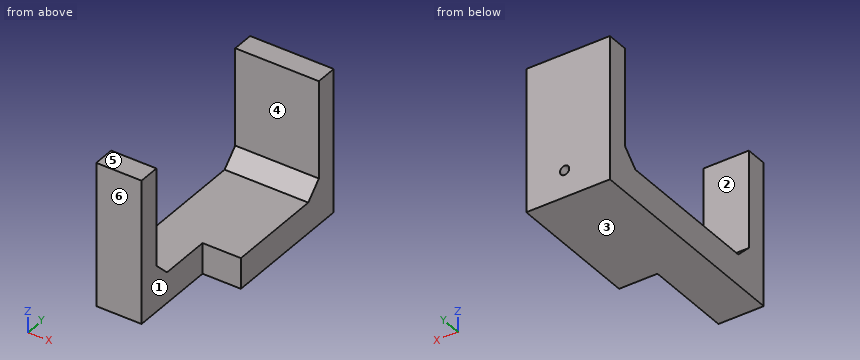
```python
from build123d import *

# Parameters (mm, degrees)
SKETCH026_W     = 10.9
SKETCH026_H     = 29
PAD009_DEPTH    = 4
SKETCH027_W     = 9
SKETCH027_H     = 14
POCKET015_DEPTH = 4.001
SKETCH028_W     = 5.9
SKETCH028_H     = 2.8
SKETCH028_W_2   = 10.9
PAD010_DEPTH    = 14.7
CHAMFER001_SIZE = 2
SKETCH033_R     = 0.6
POCKET016_DEPTH = 4


with BuildPart() as part:
    # Sketch026 (on DatumPlane) → Pad009 (new body)
    with BuildSketch(Plane.XY.offset(7)):
        with Locations((-19.95, 0)):
            Rectangle(SKETCH026_W, SKETCH026_H)
    extrude(amount=PAD009_DEPTH)

    # Sketch027 (on DatumPlane) → Pocket015 (cut, through all)
    with BuildSketch(Plane.XY.offset(11)):
        with Locations((-15, -10)):
            Rectangle(SKETCH027_W, SKETCH027_H)
    extrude(amount=-POCKET015_DEPTH, mode=Mode.SUBTRACT)

    # Sketch028 (on DatumPlane) → Pad010 (join)
    with BuildSketch(Plane.XY.offset(11)):
        with Locations((-22.45, -13.1)):
            Rectangle(SKETCH028_W, SKETCH028_H)
        with Locations((-19.95, 13.1)):
            Rectangle(SKETCH028_W_2, SKETCH028_H)
    extrude(amount=PAD010_DEPTH)

    # Chamfer001
    chamfer001_edges = [part.edges().sort_by_distance(p)[0] for p in [
        (-19.95, 11.7, 11),
        (-22.45, -11.7, 11),
    ]]
    chamfer(chamfer001_edges, length=CHAMFER001_SIZE)

    # Sketch033 (on DatumPlane) → Pocket016 (cut)
    with BuildSketch(Plane.XZ.offset(-14.5)):
        with Locations((-19.5, 10.5)):
            Circle(SKETCH033_R)
    extrude(amount=POCKET016_DEPTH, mode=Mode.SUBTRACT)


solid = part.part
```
Read the model definition and answer for the solid it produces. Units are mm, in the model's axes. Face numbers are marked on the shaded views. A direction names the side the tool comes from. Give positions to 0.01 mm unless a question says otherwise; leave off trailing zeros. Write each loop counter-clockwise with the first axis right and the second up, starting at its lowest first coordinate (ties: lowest second). Pieces come first, ordered by that corner, then holes. Notation, with made-up numbers: (-9, 37) -> (41, 37) arc R28 cw to (41, 73) -> close; hole circle Ø9 at (-10.5, -12.5). An arc over 180 degrees is marked (long way). Answer as a JSON object with one key per item and string values.
1) Section B-B on x = -22.25 is taken. Write down the section's boundary in (y, z), then the cut area to 3 significant figures.
Findings below:
{"outline": "(-14.5, 7) -> (14.5, 7) -> (14.5, 25.7) -> (11.7, 25.7) -> (11.7, 13) -> (9.7, 11) -> (-9.7, 11) -> (-11.7, 13) -> (-11.7, 25.7) -> (-14.5, 25.7) -> close", "area": "202 mm^2"}
2) For a pull along Y with two mould halves and no side action, classify the marked faces 4, 5 and 6 as pulls with the +Y half, pulls with the -Y half, needs draft (parallel to the pull), parting line crosses it, or undercut.
Findings below:
{"face 4": "undercut", "face 5": "needs draft", "face 6": "pulls with the -Y half"}
3) A tool of negligible diameter and unlimited length cuts with its end or side. For the marked faces 1, 2 and 3, from which of +Z, -Z, +X, -X, +Y, -Y can it reach the whole face along a straight path? Write none if from no direction.
Findings below:
{"face 1": "+Z, -Z, +X, -Y", "face 2": "+Z, +X, -X", "face 3": "-Z, +X, -X, +Y, -Y"}
4) Section D-D on y = -10.25 is taken. Write down the section's boundary in (x, z), then the cut area to 3 significant figures.
Findings below:
{"outline": "(-25.4, 7) -> (-19.5, 7) -> (-19.5, 11.55) -> (-25.4, 11.55) -> close", "area": "26.8 mm^2"}
5) Section C-C on z = 14 is taken. Write down the section's boundary in (x, y), then the cut area to 3 significant figures.
Findings below:
{"outline": "(-25.4, -14.5) -> (-19.5, -14.5) -> (-19.5, -11.7) -> (-25.4, -11.7) -> close; (-25.4, 11.7) -> (-14.5, 11.7) -> (-14.5, 14.5) -> (-25.4, 14.5) -> close", "area": "47.0 mm^2"}
6) Flat-ended cylindrical pins translate along their axes: pin 1 Ø5.5 at (x, z) = (-19, 22) entering from -Y; pin 2 Ø6 at (y, z) = (-10.5, 13.5) entering from +X; pin 3 Ø1.2 at (x, z) = (-18, 9.5) entering from -Y; pin 4 Ø3.5 at (x, y) = (-20, 4) entering from +Z. Find the tip coordinate at first contact, or state that the pin passes through.
Findings below:
{"pin 1": "stops at y = -14.5", "pin 2": "stops at x = -19.5", "pin 3": "stops at y = -3", "pin 4": "stops at z = 11"}
7) Section A-A on z = 11.75 is taken. Write down the section's boundary in (x, y).
Findings below:
{"outline": "(-25.4, -14.5) -> (-19.5, -14.5) -> (-19.5, -10.45) -> (-25.4, -10.45) -> close; (-25.4, 10.45) -> (-14.5, 10.45) -> (-14.5, 14.5) -> (-25.4, 14.5) -> close"}
8) Straight lines are drawn through the part: probe 1 along Y at (x, z) = (-23.5, 21.75); probe 2 along Z at (x, y) = (-19.5, 13.6); probe 3 along Z at (x, y) = (-17.5, 3). For each, find the intervals that lie inside material, in ascending order. Write a range as from..to.
Findings below:
{"probe 1": "y = -14.5..-11.7, 11.7..14.5", "probe 2": "z = 7..9.9, 11.1..25.7", "probe 3": "z = 7..11"}
